from build123d import *

# Parameters (mm, degrees)
EXTRUDE_1_DEPTH = 4
SKETCH_2_W      = 4
SKETCH_2_H      = 4
EXTRUDE_2_DEPTH = 3


with BuildPart() as part:
    # Эскиз1 → Бобышка-Вытянуть1 (new body)
    with BuildSketch(Plane(origin=(0, 0, 0), x_dir=(1, 0, 0), z_dir=(0, 1, 0))):
        Polygon((0, 0), (0, 3), (40.1, 3), (40.1, 0), (60.1, 0), (60.1, 20), (-20, 20), (-20, 0), align=None)
    extrude(amount=EXTRUDE_1_DEPTH)

    # Эскиз2 → Бобышка-Вытянуть2 (add)
    with BuildSketch(Plane.XY.offset(-3)):
        with Locations((28.1, 2)):
            Rectangle(SKETCH_2_W, SKETCH_2_H)
        with Locations((12, 2)):
            Rectangle(SKETCH_2_W, SKETCH_2_H)
    extrude(amount=EXTRUDE_2_DEPTH)


solid = part.part
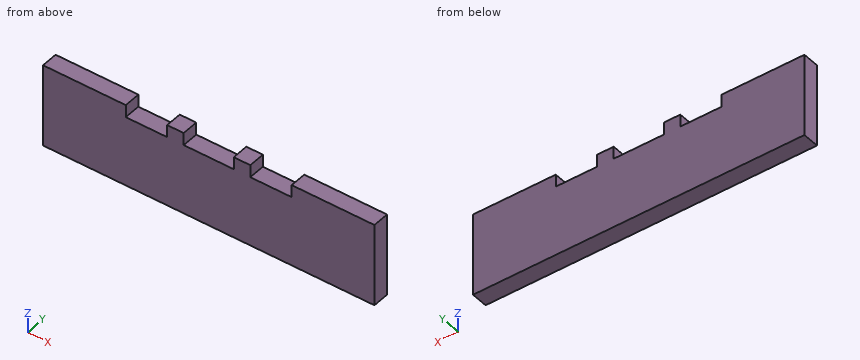
For this review, take the finished solid that the model builds, in its own axes (mm). Round coordinates to 2 decimals unless told otherwise and drop trailing zeros. Write each loop counter-clockwise with the first axis right and the second up, starting at its lowest first coordinate (ties: lowest second). Pieces come first, ordered by that corner, then holes. Notation, with made-up numbers: (-30, 84.5) - (-6, 84.5) arc R34 ccw to (-6, 121.5) - close; hole circle Ø3 at (8, 13.5). An arc over 180 degrees is marked (long way). Write item = value, one per line. Start each with the question number.
1. Consider section A-A on y = 1.9. State the section outline as (x, z) points.
2. Consider section B-B on x = 3.5. State the section outline as (y, z) points, plus the area to 3 significant figures.
3. Wall thickness on L1, parallel to X at y = 3.05, z = -2.75; L2, parallel to Z at x = 20, y = 1.55: over which ranges is each line inside the solid? List them lowest first.
4. For pin 1 Ø1.2 at (x, y) = (19.5, 3) entering from +Z, flat-tipped, find the tip position at first contact; note if it passes through.
Evaluation:
q1.outline = (-20, -20) - (60.1, -20) - (60.1, 0) - (40.1, 0) - (40.1, -3) - (30.1, -3) - (30.1, 0) - (26.1, 0) - (26.1, -3) - (14, -3) - (14, 0) - (10, 0) - (10, -3) - (0, -3) - (0, 0) - (-20, 0) - close
q2.outline = (0, -20) - (4, -20) - (4, -3) - (0, -3) - close
q2.area = 68.0 mm2
q3.L1 = -20 to 0, 10 to 14, 26.1 to 30.1, 40.1 to 60.1
q3.L2 = -20 to -3
q4.pin_1 = -3
